from build123d import *


with BuildPart() as part:
    # Sketch1 → Revolve-Thin1 (revolve)
    with BuildSketch(Plane.XY, mode=Mode.PRIVATE) as revolve_thin1_sk:
        with BuildLine():
            Line((0, 12.7), (0, 15.875))
            ThreePointArc((0, 15.875), (-1.859871939, 20.365128061), (-6.35, 22.225))
            Line((-6.35, 22.225), (-85.966255124, 22.225))
            ThreePointArc((-85.966255124, 22.225), (-92.47306886, 21.37742096), (-98.545627562, 18.89125))
            ThreePointArc((-98.545627562, 18.89125), (-104.618186264, 16.40507904), (-111.125, 15.5575))
            Line((-111.125, 15.5575), (-123.825, 15.5575))
            Line((-123.825, 15.5575), (-123.825, 16.8275))
            Line((-123.825, 16.8275), (-111.125, 16.8275))
            ThreePointArc((-111.125, 16.8275), (-104.94352695, 17.632700088), (-99.174596184, 19.9945625))
            ThreePointArc((-99.174596184, 19.9945625), (-92.798409547, 22.605042008), (-85.966255124, 23.495))
            Line((-85.966255124, 23.495), (-6.35, 23.495))
            ThreePointArc((-6.35, 23.495), (-0.961846327, 21.263153673), (1.27, 15.875))
            Line((1.27, 15.875), (1.27, 12.7))
            Line((1.27, 12.7), (0, 12.7))
        make_face()
    revolve(revolve_thin1_sk.sketch.rotate(Axis((0, 0, 0), (-1, 0, 0)), 90), axis=Axis((0, 0, 0), (-1, 0, 0)))


solid = part.part
Build history of the part. All positions in model axes, mm. A direction names the side the tool comes from. Round coordinates to 2 decimals unless told otherwise and drop trailing zeros. Write each loop counter-clockwise with the first axis right and the second up, starting at its lowest first coordinate (ties: lowest second). Pieces come first, ordered by that corner, then holes. Notation, with made-up numbers: M -25.5,78.25 L 27.5,78.25 A15 cw 27.5,82.25 Z; hole C -16.75,6 d10. An arc over 180 degrees is marked long. Answer in a Markdown table with one row per item.
1. Mould opens along Y. For faces 1 (the face through (0, -11, -7)), 2 (the face through (-45.6, 14.3, 18.64)), 3 (the face through (1.27, -11, 7)) say: +Y half, -Y half, draft (parallel to the pull), parting line (faces both ways), or undercut.
Geometry check:
| item | result |
|---|---|
| face 1 | undercut |
| face 2 | parting line |
| face 3 | draft |
2. Saw through at A-A (x = -16). List the corners of the cut face in (y, z) (3 decimals).
Geometry check:
| item | result |
|---|---|
| outline | C 0,0 d46.99; hole C 0,0 d44.45 |
3. Which spindle directions (+Z, -Z, +X, -X, +Y, -Y) get a long thin tool onto all of the face, cutting with end or side? Do faces 4 (the face through (-117.386, 16.427, 3.648)), 5 (the face through (-46.7, -15, 16.4)), 6 (the face through (-123.825, 5, 15)). Say none if no direction does.
Geometry check:
| item | result |
|---|---|
| face 4 | -X |
| face 5 | none |
| face 6 | +Z, -Z, -X, +Y, -Y |
4. Flat gauge pins, fed straight in: P1, Ø5, axis at x = -94.5, y = 2.5, coming from the -Z side; P2, Ø2, axis at y = -17.5, z = 18, coming from the -X side; P3, Ø12, axis at y = -17.5, z = 15.5, coming from the +X side; P4, Ø3, axis at x = -84.5, z = 11.5, coming from the -Y side. Where does each tip first touch, or does it go through?
Geometry check:
| item | result |
|---|---|
| P1 | z = -22.71 |
| P2 | through |
| P3 | x = 1.12 |
| P4 | y = -21.26 |
5. Probe L1, parallel to Y at x = -38.5, z = 0 (3 decimals); L2, parallel to Y at x = -118.5, z = 0; L3, parallel to Z at x = -42.5, y = 13.5. List the from-to ranges inside material, lowest first. Write a range as [from, to].
Geometry check:
| item | result |
|---|---|
| L1 | [-23.495, -22.225], [22.225, 23.495] |
| L2 | [-16.83, -15.56], [15.56, 16.83] |
| L3 | [-19.23, -17.66], [17.66, 19.23] |
